Here's how the part is built. I have some questions about the finished solid (model axes, mm). Round coordinates to 2 decimals unless told otherwise and drop trailing zeros. Loops run counter-clockwise (first coordinate to the right, second up) from the corner with the lowest first, then second, coordinate; pieces in that order, holes last. Notation, with made-up numbers: M 35.5,-13 L 83.5,-13 A26 cw 83.5,19 Z; hole C 85,54 d7. An arc over 180 degrees is marked long. Answer as CSV lines item,"result".
```python
from build123d import *

# Parameters (mm, degrees)
BOSS_EXTRUDE1_DEPTH = 10
SKETCH4_R           = 1.75
CUT_EXTRUDE2_DEPTH  = 14.957524852


with BuildPart() as part:
    # Sketch1 → Boss-Extrude1 (new body)
    with BuildSketch(Plane(origin=(0, 0, 0), x_dir=(1, 0, 0), z_dir=(0, 1, 0))):
        with BuildLine():
            Line((8.5, 4), (-5, 4))
            Line((-5, 4), (-5, -0.75))
            Line((-5, -0.75), (1.104356076, -0.75))
            Line((1.104356076, -0.75), (1.104356076, 0))
            ThreePointArc((1.104356076, 0), (2.25, 1.75), (3.395643924, 0))
            Line((3.395643924, 0), (3.395643924, -0.75))
            Line((3.395643924, -0.75), (5.104356076, -0.75))
            Line((5.104356076, -0.75), (5.104356076, 0))
            ThreePointArc((5.104356076, 0), (6.25, 1.75), (7.395643924, 0))
            Line((7.395643924, 0), (7.395643924, -0.75))
            Line((7.395643924, -0.75), (8.5, -0.75))
            Line((8.5, -0.75), (8.5, 4))
        make_face()
    extrude(amount=BOSS_EXTRUDE1_DEPTH)

    # Sketch4 → Cut-Extrude2 (cut, through all)
    with BuildSketch(Plane.XY.offset(0.75)):
        with Locations((-1.947821962, 5)):
            Circle(SKETCH4_R)
    extrude(amount=-CUT_EXTRUDE2_DEPTH, mode=Mode.SUBTRACT)


solid = part.part
```
1. We'd pull the mould along X, two halves only. Please class faces 1 (the cylindrical face through (2.22, 4.93, -1.75)), 2 (the flat face through (4, 5, 0.75)), 3 (the flat face through (8.5, 5, -2)), 4 (the cylindrical face through (6.22, 4.93, -1.75)): pulls with the +X half, pulls with the -X half, needs draft (parallel to the pull), parting line crosses it, or undercut.
Evaluation:
face 1,"undercut"
face 2,"needs draft"
face 3,"pulls with the +X half"
face 4,"undercut"
2. I want a section at A-A, the plane z = -0.5. Please give me the cut outline in (x, y).
Evaluation:
outline,"M -5,0 L 1,0 L 1,10 L -5,10 Z; M 3.5,0 L 5,0 L 5,10 L 3.5,10 Z; M 7.5,0 L 8.5,0 L 8.5,10 L 7.5,10 Z; hole C -1.95,5 d3.5"
3. For P1, Ø2, axis at x = -1.95, y = 5, coming from the -Z side, with a flat end and sliding along its axis, tell me the tip position at first contact or that it passes through.
Evaluation:
P1,"passes through"
4. I want a section at C-C, the plane x = -0.75. Please give me the cut outline in (y, z), and give its area (3 significant figures).
Evaluation:
outline,"M 0,-4 L 3.72,-4 L 3.72,0.75 L 0,0.75 Z; M 6.28,-4 L 10,-4 L 10,0.75 L 6.28,0.75 Z"
area,"35.4 mm²"
5. I want a section at B-B, the plane y = 5.5. Please give me the cut outline in (x, z).
Evaluation:
outline,"M -5,-4 L -3.62,-4 L -3.62,0.75 L -5,0.75 Z; M -0.27,-4 L 8.5,-4 L 8.5,0.75 L 7.4,0.75 L 7.4,0 A1.25 cw long 5.1,0 L 5.1,0.75 L 3.4,0.75 L 3.4,0 A1.25 cw long 1.1,0 L 1.1,0.75 L -0.27,0.75 Z"
6. If I drill on line 1 (X direction, y = 6.25, z = -0.5); line 2 (X direction, y = 4.75, z = -0.5); line 3 (Z direction, x = 2.25, y = 3.5), over which ranges is the centre line in solid material (lowest first)? Write a range as [from, to].
Evaluation:
line 1,"x = [-5, -3.17], [-0.72, 1], [3.5, 5], [7.5, 8.5]"
line 2,"x = [-5, -3.68], [-0.22, 1], [3.5, 5], [7.5, 8.5]"
line 3,"z = [-4, -1.75]"
7. I want a section at D-D, the plane z = -3.2. Please give me the cut outline in (x, y), and give its area (3 significant figures).
Evaluation:
outline,"M -5,0 L 8.5,0 L 8.5,10 L -5,10 Z; hole C -1.95,5 d3.5"
area,"125 mm²"
